Autodesk Inventor part; units mm, degrees
ref_plane "YZ Plane" through (0, 0, 0) normal (1, 0, 0) x (0, 1, 0)
ref_plane "XZ Plane" through (0, 0, 0) normal (0, 1, 0) x (-1, 0, 0)
ref_plane "XY Plane" through (0, 0, 0) normal (0, 0, 1) x (1, 0, 0)
sketch "Sketch1" plane through (0, 0, 0) normal (0, 0, 1) x (1, 0, 0)
  line L0 (0, 0) -> (-17, 0)
  line L1 (-17, 0) -> (-25.0301, -11.4681)
  line L2 (0, 0) -> (-12.6187, -18.0213)
  line L3 (0, 0) -> (22, 0) construction
  line L4 (-12.6187, -18.0213) -> (-21.1187, -18.0213)
  line L5 (-21.1187, -18.0213) -> (-25.0301, -11.4681)
  dimension "d40" = 17
  dimension "d41" = 14
  dimension "d42" = 125
  dimension "d43" = 22
  dimension "d44" = 125
  dimension "d45" = 8.5
extrude "Extrusion1" add sketch "Sketch1" along normal blind 15
shell "Shell1" thickness 0.5 removed faces 2 at (-5.6667, 0, 5) at (-9.8729, -6.0071, 0)
properties part number "metal_shielding"
Work out the finished part from the listing and answer in its coordinate system (mm). A direction names the side the tool comes from. Give positions to 0.01 mm unless a question says otherwise; leave off trailing zeros. Write each loop counter-clockwise with the first axis right and the second up, starting at its lowest first coordinate (ties: lowest second). Pieces come first, ordered by that corner, then holes. Notation, with made-up numbers: (64, 22) -> (83, 22) arc R23 ccw to (83, 49) -> close; hole circle Ø7 at (23, 11.25). An arc over 180 degrees is marked (long way). Write each question's results on one line, items separated by ' | '.
1. Straight lines are drawn through the part: L1, parallel to X at y = -16, z = 9.25; L2, parallel to Z at x = -21, y = -17; L3, parallel to Y at x = -14.25, z = 8.5. For each, find the intervals that lie inside material, in ascending order.
Data:
L1: -22.33 to -21.74, -11.81 to -11.2 | L2: 14.5 to 15 | L3: -18.02 to -17.52
2. Find section C-C on y = -16.25. Determine the outline of the cut face in (x, z).
Data:
outline: (-22.18, 0) -> (-21.59, 0) -> (-21.59, 14.5) -> (-11.99, 14.5) -> (-11.99, 0) -> (-11.38, 0) -> (-11.38, 15) -> (-22.18, 15) -> close
3. Determine the mould class of faces 1 (the flat face through (-17, -17.521, 7)), 2 (the flat face through (-13, -9, 15)), 3 (the flat face through (-17, -18.021, 7)) for opening direction Y: +Y half, -Y half, draft (parallel to the pull), parting line (faces both ways), or undercut.
Data:
face 1: undercut | face 2: draft | face 3: -Y half
4. Find section A-A on z = 6.25. Determine the outline of the cut face in (x, y), and give its area (3 significant figures).
Data:
outline: (-25.03, -11.47) -> (-21.12, -18.02) -> (-12.62, -18.02) -> (0, 0) -> (-0.61, 0) -> (-12.88, -17.52) -> (-20.83, -17.52) -> (-24.43, -11.49) -> (-16.39, 0) -> (-17, 0) -> close | area: 25.6 mm^2
5. Find section D-D on y = -2.25. Determine the outline of the cut face in (x, z), and give its area (3 significant figures).
Data:
outline: (-18.58, 0) -> (-17.97, 0) -> (-17.97, 14.5) -> (-2.19, 14.5) -> (-2.19, 0) -> (-1.58, 0) -> (-1.58, 15) -> (-18.58, 15) -> close | area: 26.2 mm^2
6. Find section B-B on x = -15.75. Determine the outline of the cut face in (y, z), and give its area (3 significant figures).
Data:
outline: (-18.02, 0) -> (-17.52, 0) -> (-17.52, 14.5) -> (0, 14.5) -> (0, 15) -> (-18.02, 15) -> close | area: 16.3 mm^2
7. Each of these flat-tipped pins is pushed along its axis until it touches: pin 1 Ø1 at (y, z) = (-10.5, 1.5) entering from -X; pin 2 Ø8 at (x, z) = (-8.5, 10) entering from +Y; pin 3 Ø2 at (y, z) = (-2, 5.5) entering from -X. Where does it stop, or does it pass through?
Data:
pin 1: x = -24.7 | pin 2: y = -5.55 | pin 3: x = -19.1
8. A tool of negligible diameter and unlimited length cuts with its end or side. For faces 4 (the flat face through (-6.66, -8.64, 7.15)), 5 (the flat face through (-13, -9, 14.5)), 6 (the flat face through (-23.047, -14.791, 7.395)), from which of +Z, -Z, +X, -X, +Y, -Y can it reach the whole face along a straight path? Write none if from no direction.
Data:
face 4: -Z, +Y | face 5: -Z | face 6: +Z, -Z, -X, -Y
